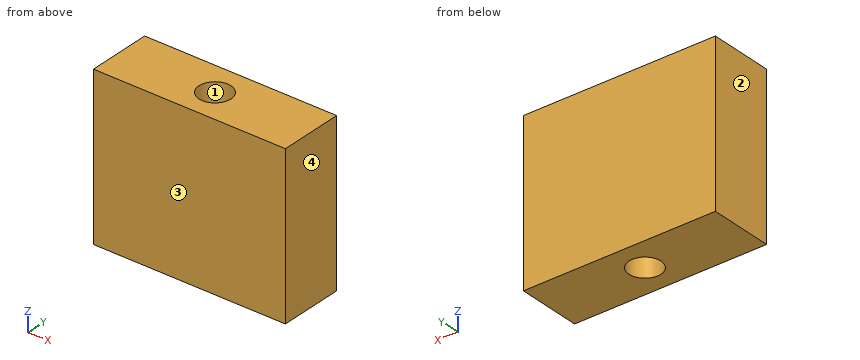
```python
from build123d import *

# Parameters (mm, degrees)
SKETCH_1_W      = 60
SKETCH_1_H      = 20
SKETCH_1_R      = 5
EXTRUDE_1_DEPTH = 25


with BuildPart() as part:
    # 草圖1 → 填料-伸長1 (new, symmetric)
    with BuildSketch(Plane.XY):
        with Locations((30, 10)):
            Rectangle(SKETCH_1_W, SKETCH_1_H)
        with Locations((30, 10)):
            Circle(SKETCH_1_R, mode=Mode.SUBTRACT)
    extrude(amount=EXTRUDE_1_DEPTH, both=True)


solid = part.part
```
Design review of the part built by this model. Coordinates are the model's own, in mm. Face numbers are marked on the shaded views. Coordinates: 2 decimals unless noted, no trailing zeros. Order: outer loops, then holes, each group sorted by start corner. A loop starts at its lowest first (then second) coordinate and runs counter-clockwise, first axis right, second up.
1) Take a section at A-A, the plane x = 30. Give the boundary of the cut face in (y, z), and give its area (3 significant figures).
2) Mouldability with a two-part tool opening along X and no side actions: class the marked faces 1, 2, 3 and 4 as +X half, -X half, draft (parallel to the pull), parting line (faces both ways), or undercut.
3) Take a section at B-B, the plane y = 10. Give the boundary of the cut face in (x, z), and give its area (3 significant figures).
4) Take a section at C-C, the plane z = -18. Give the boundary of the cut face in (x, y), and give its area (3 significant figures).
5) Wall thickness on line 1 along Y through (x, z) = (30, -1); line 2 along X through (y, z) = (7.75, -0.5); line 3 along X through (y, z) = (8.25, -20.5): over which ranges is each line inside the solid? List them lowest first.
Returned:
1. outline: (0, -25) - (5, -25) - (5, 25) - (0, 25) - close; (15, -25) - (20, -25) - (20, 25) - (15, 25) - close
1. area: 500 mm2
2. face 1: undercut
2. face 2: -X half
2. face 3: draft
2. face 4: +X half
3. outline: (0, -25) - (25, -25) - (25, 25) - (0, 25) - close; (35, -25) - (60, -25) - (60, 25) - (35, 25) - close
3. area: 2,500 mm2
4. outline: (0, 0) - (60, 0) - (60, 20) - (0, 20) - close; hole circle Ø10 at (30, 10)
4. area: 1,120 mm2
5. line 1: y = 0 to 5, 15 to 20
5. line 2: x = 0 to 25.53, 34.47 to 60
5. line 3: x = 0 to 25.32, 34.68 to 60
